The figure shows three views and two pictorial views of one solid part (mm, origin at its lowest corner). Answer the questions. Give positions to 0.01 mm unless a question says otherwise; leave off trailing zeros. Loops run counter-clockwise (first coordinate to the right, second up) from the corner with the lowest first, then second, coordinate; pieces in that order, holes last. Notation, with made-up numbers: M -28.5,79 L 27.5,79 A34 cw 27.5,115 Z; hole C 68,9 d6. An arc over 180 degrees is marked long. Answer as a JSON object with one key per item and string values. Group by question number.
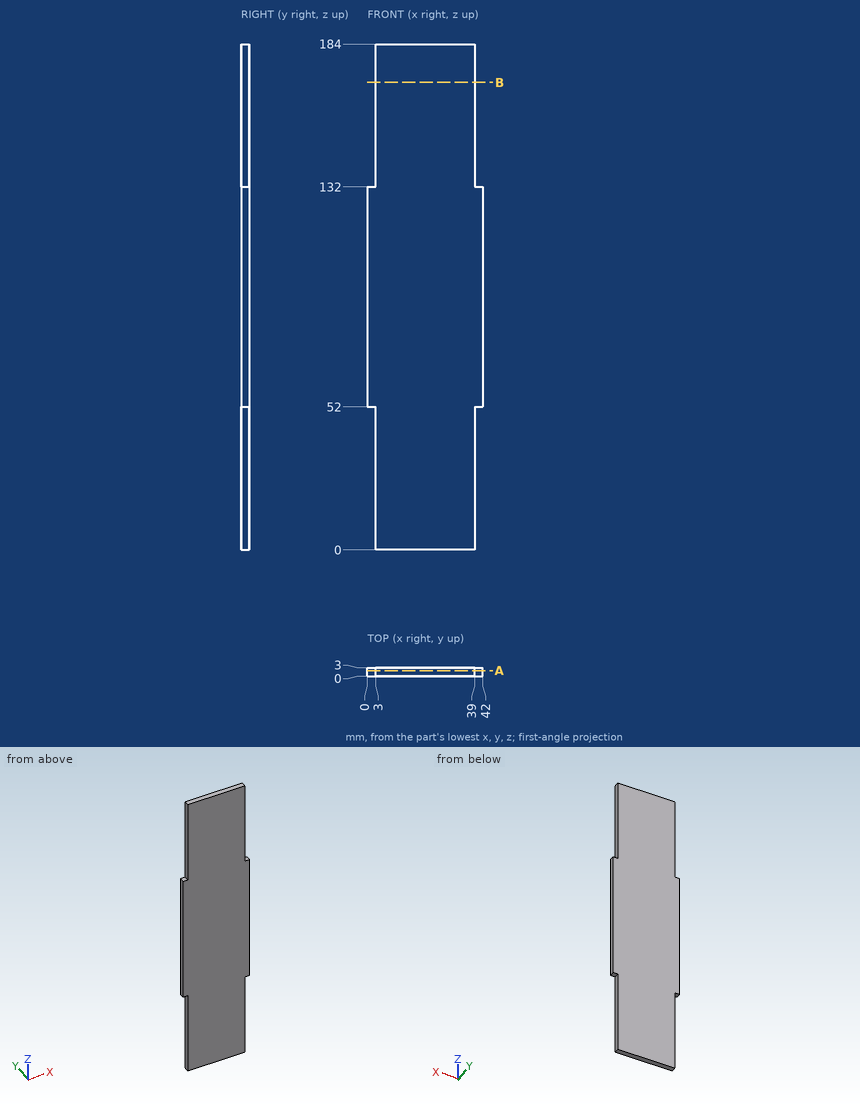
Item 1: Find the intervals of material crossed by probe 1 along X at (y, z) = (1.75, 156); probe 2 along Z at (x, y) = (2.5, 2.25), in increasing order. Write a range as [from, to].
Item 2: A cutting plane is placed at B-B (z = 170). Determine the outline of the cut face in (x, y), and give its area (3 significant figures).
Item 3: A cutting plane is placed at A-A (y = 1.95). Determine the outline of the cut face in (x, z).
Item 4: Given pin 1 Ø0.9 at (y, z) = (1, 157) entering from +X; pin 2 Ø1.5 at (y, z) = (2, 35) entering from -X; pin 3 Ø1.5 at (x, y) = (40, 2) entering from -Z, each flat-ended and moving along its own axis, determine where each tip first touches the part or whether it passes through.
The answers:
{
 "1": {"probe 1": "x = [3, 39]", "probe 2": "z = [52, 132]"},
 "2": {"outline": "M 3,0 L 39,0 L 39,3 L 3,3 Z", "area": "108 mm^2"},
 "3": {"outline": "M 0,52 L 3,52 L 3,0 L 39,0 L 39,52 L 42,52 L 42,132 L 39,132 L 39,184 L 3,184 L 3,132 L 0,132 Z"},
 "4": {"pin 1": "stops at x = 39", "pin 2": "stops at x = 3", "pin 3": "stops at z = 52"}
}
